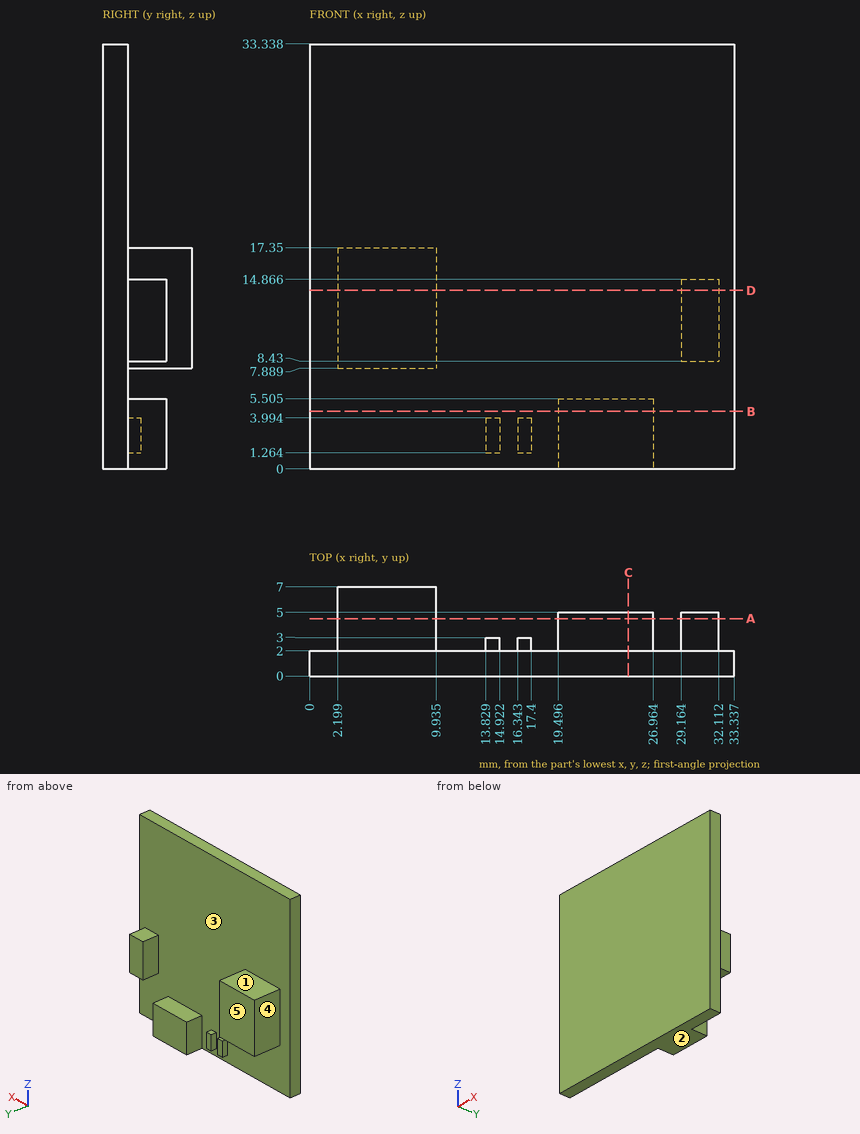
Answer from the drawing. Dimensions are ordinates in mm from the lowest x, y and z of the part. A direction names the side the tool comes from. Give positions to 0.01 mm unless a question says otherwise; leave off trailing zeros. Order: outer loops, then holes, each group sorted by start corner. A loop starts at its lowest first (then second) coordinate and runs counter-clockwise, first axis right, second up. Notation, with made-up numbers: (14, -33) - (44, -33) arc R28 cw to (44, 3) - close; hole circle Ø6 at (66.25, 75). An arc over 180 degrees is marked (long way). One line per item, written item: value. Start each with the question number.
1. Section C-C, the plane x = 25 is taken. Write down the section's boundary in (y, z) (1 decimal).
2. Each of these flat-tipped pins is pushed along its axis until it touches: pin 1 Ø0.5 at (y, z) = (2.5, 2.5) entering from -X; pin 2 Ø1.2 at (x, z) = (17, 2.5) entering from +Y; pin 3 Ø1.5 at (y, z) = (3.5, 2) entering from +X. Where does it stop, or does it pass through?
3. For a pull along X with two mould halves and no side action, classify the marked faces 3, 4 and 5 as released by +X, released by -X, zero draft, split by the parting line, or undercut.
4. Section A-A, the plane y = 4.5 is taken. Count the separate pieces of the cut face and the enclosed holes in it, then the cut area to 3 significant figures.
5. Consider line 1 (X direction, y = 2.75, z = 2) (1 decimal); line 2 (X direction, y = 2.5, z = 9) (1 decimal); line 3 (Y direction, x = 21, z = 18). Determine where each line is inside the solid, lowest interval first.
6. Section D-D, the plane z = 14 is taken. Write down the section's boundary in (x, y) (1 decimal).
7. Which of the six approach directions +Z, -Z, +X, -X, +Y, -Y give full straight-line access (tool end or side, diameter ignored) to the marked faces 1 and 2?
8. Section B-B, the plane z = 4.5 is taken. Write down the section's boundary in (x, y) (1 decimal).
Filled sheet:
1. outline: (0, 0) - (5, 0) - (5, 5.5) - (2, 5.5) - (2, 33.3) - (0, 33.3) - close
2. pin 1: x = 13.83
2. pin 2: y = 3
2. pin 3: x = 26.96
3. face 3: undercut
3. face 4: released by -X
3. face 5: zero draft
4. separate pieces: 3
4. enclosed holes: 0
4. area: 133 mm²
5. line 1: 13.8 to 14.9, 16.3 to 17.4, 19.5 to 27
5. line 2: 2.2 to 9.9, 29.2 to 32.1
5. line 3: 0 to 2
6. outline: (0, 0) - (33.3, 0) - (33.3, 2) - (32.1, 2) - (32.1, 5) - (29.2, 5) - (29.2, 2) - (9.9, 2) - (9.9, 7) - (2.2, 7) - (2.2, 2) - (0, 2) - close
7. face 1: +Z, +X, -X, +Y
7. face 2: -Z, +X, -X, +Y, -Y
8. outline: (0, 0) - (33.3, 0) - (33.3, 2) - (27, 2) - (27, 5) - (19.5, 5) - (19.5, 2) - (0, 2) - close
